Geometry check sheet. Reference: drawing and pictorial views, mm from the part's lowest x, y, z. Give positions to 0.01 mm unless a question says otherwise; leave off trailing zeros. Write each loop counter-clockwise with the first axis right and the second up, starting at its lowest first coordinate (ties: lowest second). Pieces come first, ordered by that corner, then holes.
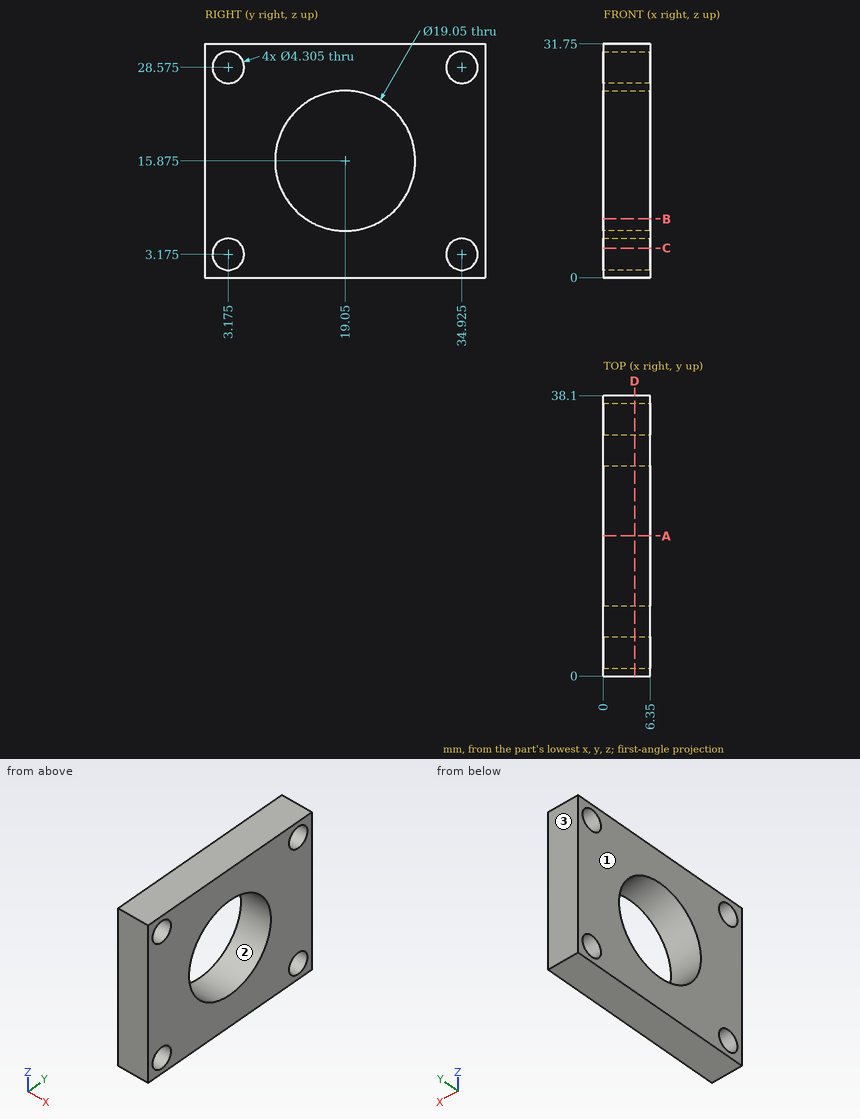
Item 1: Sectioned sample at C-C on z = 4. Record the cut outline in (x, y).
Answer key:
outline: (0, 0) - (6.35, 0) - (6.35, 1.19) - (0, 1.19) - close; (0, 5.16) - (6.35, 5.16) - (6.35, 32.94) - (0, 32.94) - close; (0, 36.91) - (6.35, 36.91) - (6.35, 38.1) - (0, 38.1) - close
Item 2: Sectioned sample at D-D on x = 4.25. State how many separate pieces and enclosed holes the cut face has.
Answer key:
separate pieces: 1
enclosed holes: 5
Item 3: Sectioned sample at A-A on y = 19.05. Record the cut outline in (x, z).
Answer key:
outline: (0, 0) - (6.35, 0) - (6.35, 6.35) - (0, 6.35) - close; (0, 25.4) - (6.35, 25.4) - (6.35, 31.75) - (0, 31.75) - close
Item 4: Release check for a two-part mould opening along Y. For the marked faces 1, 2 and 3 record: released by +Y, released by -Y, zero draft, split by the parting line, or undercut.
Answer key:
face 1: zero draft
face 2: undercut
face 3: released by +Y
Item 5: Depth check by flat-ended pin: pin 1 (6 mm diameter, centred on y = 28, z = 6.5, fed in from -X). Enter the tip coordinate at first touch or a pass-through.
Answer key:
pin 1: stops at x = 0
Item 6: Sectioned sample at B-B on z = 8. Record the cut outline in (x, y).
Answer key:
outline: (0, 0) - (6.35, 0) - (6.35, 13.69) - (0, 13.69) - close; (0, 24.41) - (6.35, 24.41) - (6.35, 38.1) - (0, 38.1) - close
Item 7: Scan lines: line 1 along Y through (x, z) = (3.75, 27); line 2 along Y through (x, z) = (2.5, 15.5); line 3 along Y through (x, z) = (4.25, 17). Record each from-to range of solid material in increasing order.
Answer key:
line 1: y = 0 to 1.71, 4.64 to 33.46, 36.39 to 38.1
line 2: y = 0 to 9.53, 28.57 to 38.1
line 3: y = 0 to 9.59, 28.51 to 38.1
